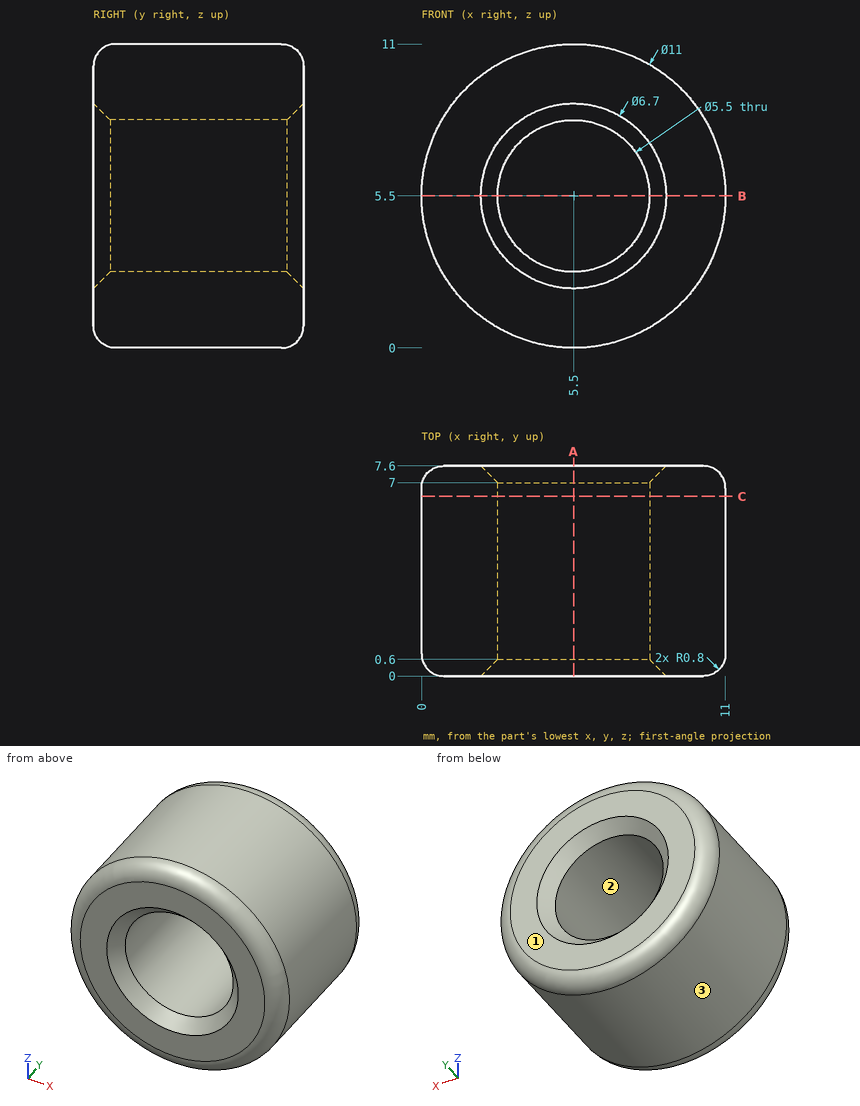
Could you check a few things on this drawing? It's one solid part, dimensions in mm from its lowest x, y, z. Coordinates: 2 decimals unless noted, no trailing zeros. Order: outer loops, then holes, each group sorted by start corner. A loop starts at its lowest first (then second) coordinate and runs counter-clockwise, first axis right, second up. Notation, with made-up numbers: (26.5, 36.5) -> (33.5, 36.5) arc R20 cw to (33.5, 47.5) -> close; hole circle Ø7 at (-33.5, 80). An arc over 180 degrees is marked (long way). One line per item, written item: value. Start each with the question number.
1) If I drill on L1, parallel to Z at x = 5.5, y = 2.5; L2, parallel to Z at x = 7, y = 5.5; L3, parallel to X at y = 4.25, z = 7.25, over which ranges is the centre line in solid material (lowest first)? Write a range as [from, to].
2) Imagine slicing it at C-C on y = 6.5. List the corners of the cut face in (x, z) for me, plus the area to 3 significant figures.
3) Imagine slicing it at B-B on z = 5.5. List the corners of the cut face in (x, y) for me.
4) I'm going to push flat-ended pins straight in: pin 1 (2 mm diameter, centred on x = 6, z = 3.5, fed in from +Y); pin 2 (3 mm diameter, centred on y = 4.5, z = 3, fed in from +X). Where does each tip first touch, or does it pass through?
5) We'd pull the mould along X, two halves only. Please class the marked faces 1, 2 and 3: +X half, -X half, draft (parallel to the pull), parting line (faces both ways), or undercut.
6) Imagine slicing it at A-A on x = 5.5. List the corners of the cut face in (y, z) for me, plus the area to 3 significant figures.
Answer list:
1. L1: z = [0, 2.75], [8.25, 11]
1. L2: z = [0.21, 3.2], [7.8, 10.79]
1. L3: x = [0.29, 3.38], [7.62, 10.71]
2. outline: circle Ø11 at (5.5, 5.5); hole circle Ø5.5 at (5.5, 5.5)
2. area: 71.3 mm2
3. outline: (0, 0.8) arc R0.8 ccw to (0.8, 0) -> (2.15, 0) -> (2.75, 0.6) -> (2.75, 7) -> (2.15, 7.6) -> (0.8, 7.6) arc R0.8 ccw to (0, 6.8) -> close; (8.25, 0.6) -> (8.85, 0) -> (10.2, 0) arc R0.8 ccw to (11, 0.8) -> (11, 6.8) arc R0.8 ccw to (10.2, 7.6) -> (8.85, 7.6) -> (8.25, 7) -> close
4. pin 1: stops at y = 7.31
4. pin 2: stops at x = 10.91
5. face 1: draft
5. face 2: undercut
5. face 3: parting line
6. outline: (0, 0.8) arc R0.8 ccw to (0.8, 0) -> (6.8, 0) arc R0.8 ccw to (7.6, 0.8) -> (7.6, 2.15) -> (7, 2.75) -> (0.6, 2.75) -> (0, 2.15) -> close; (0, 8.85) -> (0.6, 8.25) -> (7, 8.25) -> (7.6, 8.85) -> (7.6, 10.2) arc R0.8 ccw to (6.8, 11) -> (0.8, 11) arc R0.8 ccw to (0, 10.2) -> close
6. area: 40.5 mm2
